Geometry check sheet. Reference: drawing and pictorial views, mm from the part's lowest x, y, z. Give positions to 0.01 mm unless a question says otherwise; leave off trailing zeros. Loops run counter-clockwise (first coordinate to the right, second up) from the corner with the lowest first, then second, coordinate; pieces in that order, holes last. Notation, with made-up numbers: (-37.5, -1.5) -> (-31.5, -1.5) arc R23 cw to (-31.5, 7.5) -> close; hole circle Ø6 at (3.5, 30). An arc over 180 degrees is marked (long way). Write each question's results on one line, items separated by ' | '. Start each with the question number.
1. Cross-section at B-B on x = 101.5. Record the boundary of the cut face in (y, z), and give its area (3 significant figures).
2. Cross-section at A-A on y = 72.5. Record the boundary of the cut face in (x, z), and give its area (3 significant figures).
3. Material ranges on L1, parallel to X at y = 44.5, z = 3.5; L2, parallel to Y at x = 101.5, z = 2.5; L3, parallel to Y at x = 106.5, z = 7.5, recorded low to high. Write a range as from..to.
4. Cross-section at C-C on z = 6. Record the boundary of the cut face in (x, y), and give its area (3 significant figures).
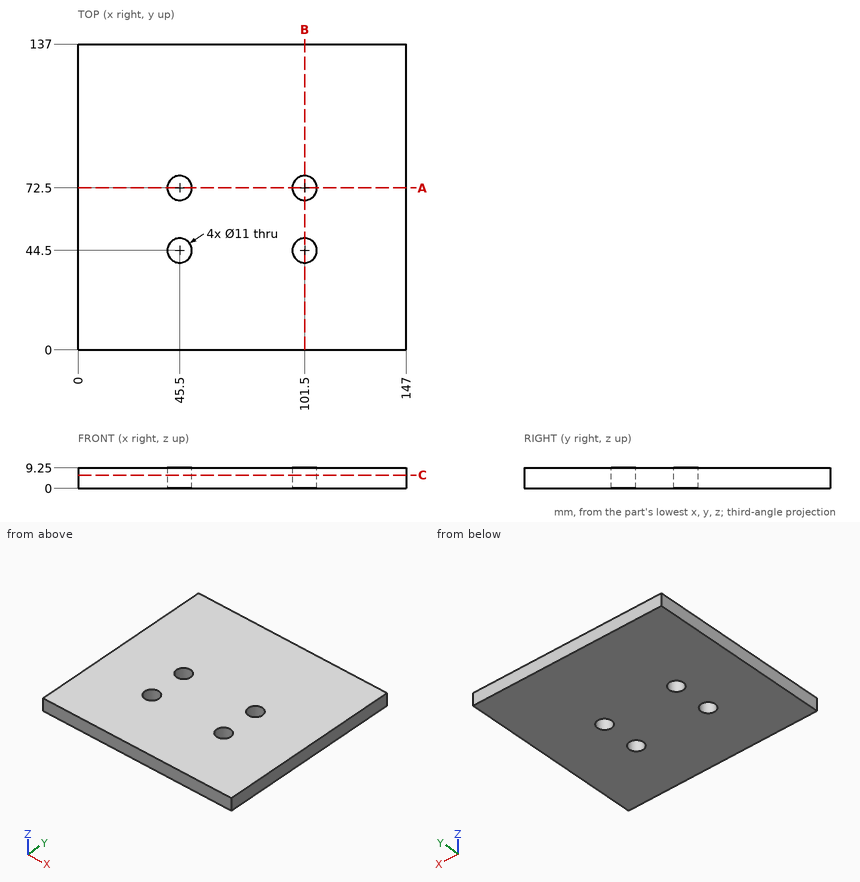
Geometry says:
1) outline: (0, 0) -> (39, 0) -> (39, 9.25) -> (0, 9.25) -> close; (50, 0) -> (67, 0) -> (67, 9.25) -> (50, 9.25) -> close; (78, 0) -> (137, 0) -> (137, 9.25) -> (78, 9.25) -> close | area: 1,060 mm^2
2) outline: (0, 0) -> (40, 0) -> (40, 9.25) -> (0, 9.25) -> close; (51, 0) -> (96, 0) -> (96, 9.25) -> (51, 9.25) -> close; (107, 0) -> (147, 0) -> (147, 9.25) -> (107, 9.25) -> close | area: 1,160 mm^2
3) L1: 0..40, 51..96, 107..147 | L2: 0..39, 50..67, 78..137 | L3: 0..42.21, 46.79..70.21, 74.79..137
4) outline: (0, 0) -> (147, 0) -> (147, 137) -> (0, 137) -> close; hole circle Ø11 at (45.5, 44.5); hole circle Ø11 at (45.5, 72.5); hole circle Ø11 at (101.5, 44.5); hole circle Ø11 at (101.5, 72.5) | area: 19,800 mm^2
